For this review, take the finished solid that the model builds, in its own axes (mm). Give positions to 0.01 mm unless a question says otherwise; leave off trailing zeros.
```python
from build123d import *

# Parameters (mm, degrees)
F3_W           = 300
F3_H           = 418
F0_DEPTH       = 18
F2_D           = 7
F2_CSINK_D     = 12.5
F2_CSINK_ANGLE = 90


with BuildPart() as f0:
    # F3 (on Top) → F0 (new body)
    with BuildSketch(Plane.XY):
        with Locations((150, 209)):
            Rectangle(F3_W, F3_H)
    extrude(amount=F0_DEPTH)

    # F2 (through all)
    with Locations(Plane.XY.offset(18)):
        with Locations((9, 50), (291, 50), (9, 300), (291, 300), (50, 409), (250, 409)):
            CounterSinkHole(F2_D / 2, F2_CSINK_D / 2, counter_sink_angle=F2_CSINK_ANGLE)


solid = f0.part
```
Q1. Mouldability with a two-part tool opening along X and no side actions: class faces 1 (the flat face through (300, 206, 9)), 2 (the conical face through (50.788, 405.453, 15.384)), 3 (the flat face through (148, 0, 9)) as +X half, -X half, draft (parallel to the pull), parting line (faces both ways), or undercut.
Answers:
face 1: +X half
face 2: undercut
face 3: draft
Q2. For pin 1 Ø8 at (x, y) = (9, 300) entering from +Z, flat-tipped, find the tip position at first contact; note if it passes through.
Answers:
pin 1: stops at z = 15.75
Q3. For probe 1 along X at (y, z) = (409, 10.5); probe 2 along Y at (x, z) = (9, 8.25); probe 3 along X at (y, z) = (50, 7.5), list the stretches that pass through material, from the lowest coordinate up.
Answers:
probe 1: x = 0 to 46.5, 53.5 to 246.5, 253.5 to 300
probe 2: y = 0 to 46.5, 53.5 to 296.5, 303.5 to 418
probe 3: x = 0 to 5.5, 12.5 to 287.5, 294.5 to 300
